```python
from build123d import *

# Parameters (mm, degrees)
SKETCH1_R                = 200
BOSS_EXTRUDE1_DEPTH      = 15
BOSS_EXTRUDE2_DEPTH      = 200
CUT_EXTRUDE1_DEPTH       = 286.087705803
CUT_EXTRUDE1_DEPTH_BACK  = 286.087705803
SKETCH3_R                = 85
CUT_EXTRUDE2_DEPTH       = 451.079120005
CUT_EXTRUDE2_DEPTH_BACK  = 451.079120005
SKETCH4_R                = 11
CUT_EXTRUDE3_DEPTH       = 451.079120105
CUT_EXTRUDE3_DEPTH_BACK  = 110
CUT_EXTRUDE4_DEPTH       = 110
BOSS_EXTRUDE3_DEPTH      = 200
CUT_EXTRUDE5_DEPTH       = 286.087705815
CUT_EXTRUDE5_DEPTH_BACK  = 286.087705815
SKETCH7_OUTSIDE_W        = 515.59
SKETCH7_OUTSIDE_H        = 515.59
SKETCH7_OUTSIDE_R        = 200
SKETCH9_R                = 4
BOSS_EXTRUDE4_DEPTH      = 220
CUT_EXTRUDE6_DEPTH       = 190
SKETCH11_R               = 3
CUT_EXTRUDE7_DEPTH       = 486.974499745
CUT_EXTRUDE8_DEPTH       = 302.61434707
CUT_EXTRUDE8_DEPTH_BACK  = 302.61434707
BOSS_EXTRUDE5_DEPTH      = 150
CUT_EXTRUDE9_DEPTH       = 262.287608345
CUT_EXTRUDE9_DEPTH_BACK  = 262.287608345
CUT_EXTRUDE10_DEPTH      = 259.795285906
CUT_EXTRUDE10_DEPTH_BACK = 259.795285906
SKETCH18_R               = 85
CUT_EXTRUDE11_START      = -15
CUT_EXTRUDE11_DEPTH      = 35
SKETCH20_R               = 2.75
CUT_EXTRUDE12_DEPTH      = 268.341007469
CUT_EXTRUDE13_DEPTH      = 3
CUT_EXTRUDE14_DEPTH      = 3
LPATTERN1_COUNT          = 3
LPATTERN1_PITCH          = 30
SKETCH23_R               = 1.65
CUT_EXTRUDE15_DEPTH      = 20
LPATTERN2_COUNT          = 3
LPATTERN2_PITCH          = 30
CUT_EXTRUDE16_DEPTH      = 3


# Read off the part's stored shape, not the designer's step: Cut-Extrude11
with BuildPart() as part:
    # Sketch1 → Boss-Extrude1 (new body)
    with BuildSketch(Plane(origin=(0, 0, 0), x_dir=(1, 0, 0), z_dir=(0, 1, 0))):
        with Locations(Location((0, 0, 0), (0, 0, 270))):
            Circle(SKETCH1_R)
    extrude(amount=BOSS_EXTRUDE1_DEPTH)

    # Sketch2 → Boss-Extrude2 (add, symmetric)
    with BuildSketch(Plane.XY):
        Polygon((-25, 50.707142143), (25, 50.707142143), (60, 15), (-60, 15), align=None)
    extrude(amount=BOSS_EXTRUDE2_DEPTH, both=True)

    # Sketch3 → Cut-Extrude1 (cut, two sides: drawn at the far end of the back side and taken through both)
    with BuildSketch(Plane(origin=(0, 15, 0), x_dir=(1, 0, 0), z_dir=(0, 1, 0)).offset(-CUT_EXTRUDE1_DEPTH_BACK)):
        with Locations(Location((0, 0, 0), (0, 0, 270))):
            Circle(SKETCH3_R)
    extrude(amount=CUT_EXTRUDE1_DEPTH + CUT_EXTRUDE1_DEPTH_BACK, mode=Mode.SUBTRACT)

    # Sketch4 → Cut-Extrude2 (cut, two sides: drawn at the far end of the back side and taken through both)
    with BuildSketch(Plane(origin=(0, 0, -200), x_dir=(-1, 0, 0), z_dir=(0, 0, -1)).offset(-CUT_EXTRUDE2_DEPTH_BACK)):
        with Locations((0, 29)):
            Circle(SKETCH4_R)
    extrude(amount=CUT_EXTRUDE2_DEPTH + CUT_EXTRUDE2_DEPTH_BACK, mode=Mode.SUBTRACT)

    # Sketch5 → Cut-Extrude3 (cut, two sides: drawn at the far end of the back side and taken through both)
    with BuildSketch(Plane.XY.offset(200).offset(-CUT_EXTRUDE3_DEPTH_BACK)):
        Polygon((-25, 50.707142143), (25, 50.707142143), (50.198039412, 25), (25, 25), (25, 15), (-25, 15), (-25, 25), (-50.198039412, 25), align=None)
    extrude(amount=CUT_EXTRUDE3_DEPTH + CUT_EXTRUDE3_DEPTH_BACK, mode=Mode.SUBTRACT)

    # Sketch6 → Cut-Extrude4 (cut)
    with BuildSketch(Plane(origin=(0, 0, -200), x_dir=(-1, 0, 0), z_dir=(0, 0, -1))):
        Polygon((-25, 50.707142143), (25, 50.707142143), (50.198039412, 25), (25, 25), (25, 15), (-25, 15), (-25, 25), (-50.198039412, 25), align=None)
    extrude(amount=-CUT_EXTRUDE4_DEPTH, mode=Mode.SUBTRACT)

    # Sketch8 → Boss-Extrude3 (add, symmetric)
    with BuildSketch(Plane(origin=(0, 0, 0), x_dir=(0, 0, -1), z_dir=(1, 0, 0))):
        Polygon((0, 15), (-20, 15), (-10, 35.712315177), (10, 35.712315177), (20, 15), align=None)
    extrude(amount=BOSS_EXTRUDE3_DEPTH, both=True)

    # Sketch7 outside → Cut-Extrude5 (cut, two sides: drawn at the far end of the back side and taken through both)
    with BuildSketch(Plane(origin=(0, 15, 0), x_dir=(1, 0, 0), z_dir=(0, 1, 0)).offset(-CUT_EXTRUDE5_DEPTH_BACK)):
        Rectangle(SKETCH7_OUTSIDE_W, SKETCH7_OUTSIDE_H)
        with Locations(Location((0, 0, 0), (0, 0, 97.180755781))):
            Circle(SKETCH7_OUTSIDE_R, mode=Mode.SUBTRACT)
    extrude(amount=CUT_EXTRUDE5_DEPTH + CUT_EXTRUDE5_DEPTH_BACK, mode=Mode.SUBTRACT)

    # Sketch9 → Boss-Extrude4 (add, symmetric)
    with BuildSketch(Plane(origin=(0, 0, 0), x_dir=(0, 0, -1), z_dir=(1, 0, 0))):
        with Locations(Location((0, 29, 0), (0, 0, 180))):
            Circle(SKETCH9_R)
    extrude(amount=BOSS_EXTRUDE4_DEPTH, both=True)

    # Sketch10 → Cut-Extrude6 (cut, symmetric)
    with BuildSketch(Plane(origin=(0, 0, 0), x_dir=(0, 0, -1), z_dir=(1, 0, 0))):
        Polygon((-20, 15), (20, 15), (10, 35.712315177), (-10, 35.712315177), align=None)
    extrude(amount=CUT_EXTRUDE6_DEPTH, both=True, mode=Mode.SUBTRACT)

    # Sketch11 → Cut-Extrude7 (cut, through all)
    with BuildSketch(Plane.ZY.offset(220)):
        with Locations((0, 29)):
            Circle(SKETCH11_R)
    extrude(amount=-CUT_EXTRUDE7_DEPTH, mode=Mode.SUBTRACT)

    # Sketch14 → Cut-Extrude8 (cut, two sides: drawn at the far end of the back side and taken through both)
    with BuildSketch(Plane(origin=(0, 0, 0), x_dir=(1, 0, 0), z_dir=(0, 1, 0)).offset(-CUT_EXTRUDE8_DEPTH_BACK)):
        Polygon((-80, 28.722813233), (-80, 204.683452683), (-270.013244013, 28.722813233), (-103.583737584, -216.10995611), (187.046893047, -216.10995611), (266.535612536, 150.034958035), (80, 209.154693155), (80, 28.722813233), align=None)
    extrude(amount=CUT_EXTRUDE8_DEPTH + CUT_EXTRUDE8_DEPTH_BACK, mode=Mode.SUBTRACT)

    # Sketch16 → Boss-Extrude5 (add, symmetric)
    with BuildSketch(Plane(origin=(0, 0, -90), x_dir=(-1, 0, 0), z_dir=(0, 0, -1))):
        Polygon((-80, 15), (-80, 35), (-70, 35), (-70, 25), (-60.807611845, 15), (-60.807611845, 0), (-80, 0), (-80, 4.5), (-90, 4.5), (-90, 10.5), (-80, 10.5), align=None)
        Polygon((80, 15), (80, 35), (70, 35), (70, 25), (60.807611845, 15), (60.807611845, 0), (80, 0), (80, 4.5), (90, 4.5), (90, 10.5), (80, 10.5), align=None)
    extrude(amount=BOSS_EXTRUDE5_DEPTH, both=True)

    # Sketch17 → Cut-Extrude9 (cut, two sides: drawn at the far end of the back side and taken through both)
    with BuildSketch(Plane(origin=(0, 0, 0), x_dir=(1, 0, 0), z_dir=(0, 1, 0)).offset(-CUT_EXTRUDE9_DEPTH_BACK)):
        Polygon((-80, 28.722813233), (-99.608008808, 28.722813233), (-99.608008808, -74.271563426), (112.245925984, -74.271563426), (112.245925984, 0), (109.222119936, 28.722813233), (80, 28.722813233), align=None)
    extrude(amount=CUT_EXTRUDE9_DEPTH + CUT_EXTRUDE9_DEPTH_BACK, mode=Mode.SUBTRACT)

    # Sketch18 → Cut-Extrude10 (cut, two sides: drawn at the far end of the back side and taken through both)
    with BuildSketch(Plane(origin=(0, 15, 0), x_dir=(1, 0, 0), z_dir=(0, 1, 0)).offset(-CUT_EXTRUDE10_DEPTH_BACK)):
        Circle(SKETCH18_R)
    extrude(amount=CUT_EXTRUDE10_DEPTH + CUT_EXTRUDE10_DEPTH_BACK, mode=Mode.SUBTRACT)

    # Cut-Extrude11 outline → Cut-Extrude11 (cut)
    with BuildSketch(Plane(origin=(0, 15, 0), x_dir=(1, 0, 0), z_dir=(0, 1, 0)).offset(CUT_EXTRUDE11_START)):
        with BuildLine():
            Line((60.807611845, 240), (60.807611845, 190.531977216))
            ThreePointArc((60.807611845, 190.531977216), (75.639228606, 185.145097413), (90, 178.605710995))
            Line((90, 178.605710995), (90, 240))
            Line((90, 240), (60.807611845, 240))
        make_face()
        with BuildLine():
            Line((-60.807611845, 190.531977216), (-60.807611845, 240))
            Line((-60.807611845, 240), (-90, 240))
            Line((-90, 240), (-90, 178.605710995))
            ThreePointArc((-90, 178.605710995), (-75.639228606, 185.145097413), (-60.807611845, 190.531977216))
        make_face()
    extrude(amount=CUT_EXTRUDE11_DEPTH, mode=Mode.SUBTRACT)

    # Sketch20 → Cut-Extrude12 (cut, through all)
    with BuildSketch(Plane.ZY.offset(80)):
        with Locations((-163.303027798, 30)):
            Circle(SKETCH20_R)
        with Locations((-103.303027798, 30)):
            Circle(SKETCH20_R)
        with Locations((-133.303027798, 30)):
            Circle(SKETCH20_R)
    extrude(amount=-CUT_EXTRUDE12_DEPTH, mode=Mode.SUBTRACT)

    # Sketch21 → Cut-Extrude13 (cut)
    with BuildSketch(Plane(origin=(-70, 0, 0), x_dir=(0, 0, -1), z_dir=(1, 0, 0))):
        Polygon((100.935891695, 34.1), (98.568755591, 30), (100.935891695, 25.9), (105.670163902, 25.9), (108.037300006, 30), (105.670163902, 34.1), (103.303027798, 34.1), align=None)
    cut_extrude13 = extrude(amount=-CUT_EXTRUDE13_DEPTH, mode=Mode.SUBTRACT)

    # Sketch22 → Cut-Extrude14 (cut)
    with BuildSketch(Plane.ZY.offset(-70)):
        Polygon((-163.303027798, 34.1), (-160.933027798, 34.1), (-158.565891695, 30), (-160.933027798, 25.9), (-163.303027798, 25.9), (-165.673027798, 25.9), (-168.040163902, 30), (-165.673027798, 34.1), align=None)
    cut_extrude14 = extrude(amount=-CUT_EXTRUDE14_DEPTH, mode=Mode.SUBTRACT)

    # LPattern1: Cut-Extrude14 ×3
    with Locations(*[(0, 0, i * LPATTERN1_PITCH) for i in range(1, LPATTERN1_COUNT)]):
        add(cut_extrude14, mode=Mode.SUBTRACT)

    # Sketch23 → Cut-Extrude15 (cut)
    with BuildSketch(Plane(origin=(0, 15, 0), x_dir=(1, 0, 0), z_dir=(0, 1, 0))):
        with Locations(Location((19.5, 152.65, 0), (0, 0, 270))):
            Circle(SKETCH23_R)
        with Locations(Location((-19.5, 152.65, 0), (0, 0, 270))):
            Circle(SKETCH23_R)
        with Locations(Location((-19.5, 190.65, 0), (0, 0, 270))):
            Circle(SKETCH23_R)
        with Locations(Location((19.5, 190.65, 0), (0, 0, 270))):
            Circle(SKETCH23_R)
    extrude(amount=-CUT_EXTRUDE15_DEPTH, mode=Mode.SUBTRACT)

    # LPattern2: Cut-Extrude13 ×3
    with Locations(*[(0, 0, -i * LPATTERN2_PITCH) for i in range(1, LPATTERN2_COUNT)]):
        add(cut_extrude13, mode=Mode.SUBTRACT)

    # Sketch24 → Cut-Extrude16 (cut)
    with BuildSketch(Plane.XZ):
        Polygon((-19.5, -187.8), (-17.854551733, -187.8), (-16.209103466, -190.65), (-17.854551733, -193.5), (-21.145448267, -193.5), (-22.790896534, -190.65), (-21.145448267, -187.8), align=None)
        Polygon((-19.5, -149.8), (-17.854551733, -149.8), (-16.209103466, -152.65), (-17.854551733, -155.5), (-21.145448267, -155.5), (-22.790896534, -152.65), (-21.145448267, -149.8), align=None)
        Polygon((19.5, -149.8), (21.145448267, -149.8), (22.790896534, -152.65), (21.145448267, -155.5), (17.854551733, -155.5), (16.209103466, -152.65), (17.854551733, -149.8), align=None)
        Polygon((19.5, -187.8), (21.145448267, -187.8), (22.790896713, -190.649999897), (21.145448624, -193.5), (17.85455209, -193.5), (16.209103644, -190.650000103), (17.854551733, -187.8), align=None)
    extrude(amount=-CUT_EXTRUDE16_DEPTH, mode=Mode.SUBTRACT)


solid = part.part
```
Verification items for the finished model (mm, model axes). A direction names the side the tool comes from. Give positions to 0.01 mm unless a question says otherwise; leave off trailing zeros. Order: outer loops, then holes, each group sorted by start corner. A loop starts at its lowest first (then second) coordinate and runs counter-clockwise, first axis right, second up. Notation, with made-up numbers: (61, 29.25) -> (115, 29.25) arc R22 ccw to (115, 66.25) -> close; hole circle Ø4 at (46, 81.5). An arc over 180 degrees is marked (long way). One line per item, written item: value.
(1) Scan lines: line 1 along X through (y, z) = (34.5, -43.5); line 2 along Y through (x, z) = (-60.5, -109.5); line 3 along Y through (x, z) = (66.5, -178). Record each from-to range of solid material in increasing order. Write a range as [from, to].
Final values:
line 1: [-80, -73.03], [73.03, 80]
line 2: [0, 15]
line 3: [0, 21.19]
(2) Sectioned sample at A-A on z = -79. Record the cut outline in (x, y), then the cut area to 3 significant figures.
Final values:
outline: (-90, 4.5) -> (-80, 4.5) -> (-80, 0) -> (-31.37, 0) -> (-31.37, 44.21) -> (-60, 15) -> (-60.81, 15) -> (-70, 25) -> (-70, 35) -> (-80, 35) -> (-80, 10.5) -> (-90, 10.5) -> close; (31.37, 0) -> (80, 0) -> (80, 4.5) -> (90, 4.5) -> (90, 10.5) -> (80, 10.5) -> (80, 35) -> (70, 35) -> (70, 25) -> (60.81, 15) -> (60, 15) -> (31.37, 44.21) -> close
area: 2,910 mm^2
(3) Tool access check on faces 1 (the face through (-50.52, 24.67, -125.97)), 2 (the face through (-21, 3, -189)), 3 (the face through (85, 10.5, -105)), 4 (the face through (25, 20, -145)). Record the directions out of +Z, -Z, +X, -X, +Y, -Y that give a thin tool (end or side, any length) a straight path to the whole face; none if there is none.
Final values:
face 1: +Z, -Z, +Y
face 2: -Y
face 3: +Z, -Z, +X, +Y
face 4: -Z, +Y
(4) Sectioned sample at B-B on x = 40.5. Record the cut outline in (y, z).
Final values:
outline: (0, -195.86) -> (25, -195.86) -> (25, -90) -> (34.89, -90) -> (34.89, -74.73) -> (0, -74.73) -> close
(5) Sectioned sample at C-C on y = 43. Record the cut outline in (x, z), then the cut area to 3 significant figures.
Final values:
outline: (-32.55, -90) -> (32.55, -90) -> (32.55, -78.52) arc R85 cw to (-32.55, -78.52) -> close
area: 464 mm^2
(6) Gauge pin test, flat ends, axial feed: pin 1 (7 mm diameter, centred on y = 30, z = -133.3, fed in from -X); pin 2 (11 mm diameter, centred on x = -85, z = -91.5, fed in from +Y); pin 3 (4 mm diameter, centred on y = 29.5, z = -48.5, fed in from +X); pin 4 (5 mm diameter, centred on x = 71.5, y = 39, fed in from +Z). Record the tip position at first contact, or that the pin passes through.
Final values:
pin 1: x = -80
pin 2: y = 35
pin 3: x = 80
pin 4: through
(7) Draft check along X on faces 5 (the face through (85, 4.5, -105)), 6 (the face through (70, 30, -117)). Enter one of: pulls with the +X half, pulls with the -X half, needs draft (parallel to the pull), parting line crosses it, or undercut.
Final values:
face 5: needs draft
face 6: undercut
